from build123d import *

# Parameters (mm, degrees)
EXTRUDE1_DEPTH  = 400
SKETCH2_R       = 3
EXTRUDE2_DEPTH  = 3.5
SKETCH_R        = 1.75
EXTRUDE3_DEPTH  = 7.5
LPATTERN1_COUNT = 40
LPATTERN1_PITCH = 20
CHAMFER1_SIZE   = 0.3


with BuildPart() as part:
    # Sketch1 → Extrude1 (new body)
    with BuildSketch(Plane.XY):
        with BuildLine():
            Line((-4.5, -3.25), (4.5, -3.25))
            Line((4.5, -3.25), (4.5, 0.45))
            ThreePointArc((4.5, 0.45), (3.887627564, 0.659430585), (3.531754163, 1.2))
            Line((3.531754163, 1.2), (3.4, 1.2))
            Line((3.4, 1.2), (3.4, 1.7))
            Line((3.4, 1.7), (3.531754163, 1.7))
            ThreePointArc((3.531754163, 1.7), (3.887627564, 2.240569415), (4.5, 2.45))
            Line((4.5, 2.45), (4.5, 3.25))
            Line((4.5, 3.25), (-4.5, 3.25))
            Line((-4.5, 3.25), (-4.5, 2.45))
            ThreePointArc((-4.5, 2.45), (-3.887627564, 2.240569415), (-3.531754163, 1.7))
            Line((-3.531754163, 1.7), (-3.4, 1.7))
            Line((-3.4, 1.7), (-3.4, 1.2))
            Line((-3.4, 1.2), (-3.531754163, 1.2))
            ThreePointArc((-3.531754163, 1.2), (-3.887627564, 0.659430585), (-4.5, 0.45))
            Line((-4.5, 0.45), (-4.5, -3.25))
        make_face()
    extrude(amount=EXTRUDE1_DEPTH)

    # Sketch2 → Extrude2 (cut)
    with BuildSketch(Plane(origin=(0, 3.25, 0), x_dir=(1, 0, 0), z_dir=(0, 1, 0))):
        with Locations((0, -5)):
            Circle(SKETCH2_R)
    extrude2 = extrude(amount=-EXTRUDE2_DEPTH, mode=Mode.SUBTRACT)

    # Sketch → Extrude3 (cut, through all)
    with BuildSketch(Plane(origin=(0, 3.25, 0), x_dir=(1, 0, 0), z_dir=(0, 1, 0))):
        with Locations((0, -5)):
            Circle(SKETCH_R)
    extrude3 = extrude(amount=-EXTRUDE3_DEPTH, mode=Mode.SUBTRACT)

    # LPattern1: Extrude2, Extrude3 ×40
    with Locations(*[(0, 0, i * LPATTERN1_PITCH) for i in range(1, LPATTERN1_COUNT)]):
        add(extrude2, mode=Mode.SUBTRACT)
        add(extrude3, mode=Mode.SUBTRACT)

    # Chamfer1
    chamfer1_edges = [part.edges().sort_by_distance(p)[0] for p in [
        (-4.5, 3.25, 200),
        (4.5, 3.25, 200),
    ]]
    chamfer(chamfer1_edges, length=CHAMFER1_SIZE)


solid = part.part
The listing builds one solid part. Answer for the finished solid, in the listing's coordinates (mm). Round coordinates to 2 decimals unless told otherwise and drop trailing zeros. Write each loop counter-clockwise with the first axis right and the second up, starting at its lowest first coordinate (ties: lowest second). Pieces come first, ordered by that corner, then holes. Notation, with made-up numbers: (73, 55) - (129, 55) arc R22 ccw to (129, 64) - close; hole circle Ø2 at (54, 39.5). An arc over 180 degrees is marked (long way). Use one line per item in the form item = value. Start each with the question number.
Item 1: A flat-ended cylindrical pin translates along its axis: pin 1 Ø5 at (x, z) = (0, 225) entering from +Y. Find the tip coordinate at first contact, or state that the pin passes through.
Item 2: A cutting plane is placed at A-A (z = 357). Write down the section's boundary in (x, y), plus the area to 3 significant figures.
Item 3: Find the intervals of material crossed by line 1 (X direction, y = -2.2, z = 45); line 2 (X direction, y = 1.95, z = 265); line 3 (Y direction, x = -3.5, z = 120), in increasing order. Write a range as [from, to].
The answers:
q1.pin_1 = -0.25
q2.outline = (-4.5, -3.25) - (4.5, -3.25) - (4.5, 0.45) arc R1 cw to (3.53, 1.2) - (3.4, 1.2) - (3.4, 1.7) - (3.53, 1.7) arc R1 cw to (4.5, 2.45) - (4.5, 2.95) - (4.2, 3.25) - (-4.2, 3.25) - (-4.5, 2.95) - (-4.5, 2.45) arc R1 cw to (-3.53, 1.7) - (-3.4, 1.7) - (-3.4, 1.2) - (-3.53, 1.2) arc R1 cw to (-4.5, 0.45) - close
q2.area = 55.2 mm^2
q3.line_1 = [-4.5, -1.75], [1.75, 4.5]
q3.line_2 = [-3.63, -3], [3, 3.63]
q3.line_3 = [-3.25, 1.2], [1.7, 3.25]
